Can you work these out from the drawing? Everything is in mm from the part's minimum corner. Give positions to 0.01 mm unless a question says otherwise; leave off trailing zeros. Order: outer loops, then holes, each group sorted by start corner. A loop starts at its lowest first (then second) coordinate and runs counter-clockwise, first axis right, second up. Notation, with made-up numbers: (8, 16.25) - (52, 16.25) arc R12 cw to (52, 36.25) - close; hole circle Ø4 at (13.5, 3.5). An arc over 180 degrees is marked (long way). Answer as a JSON object with one key per item and string values.
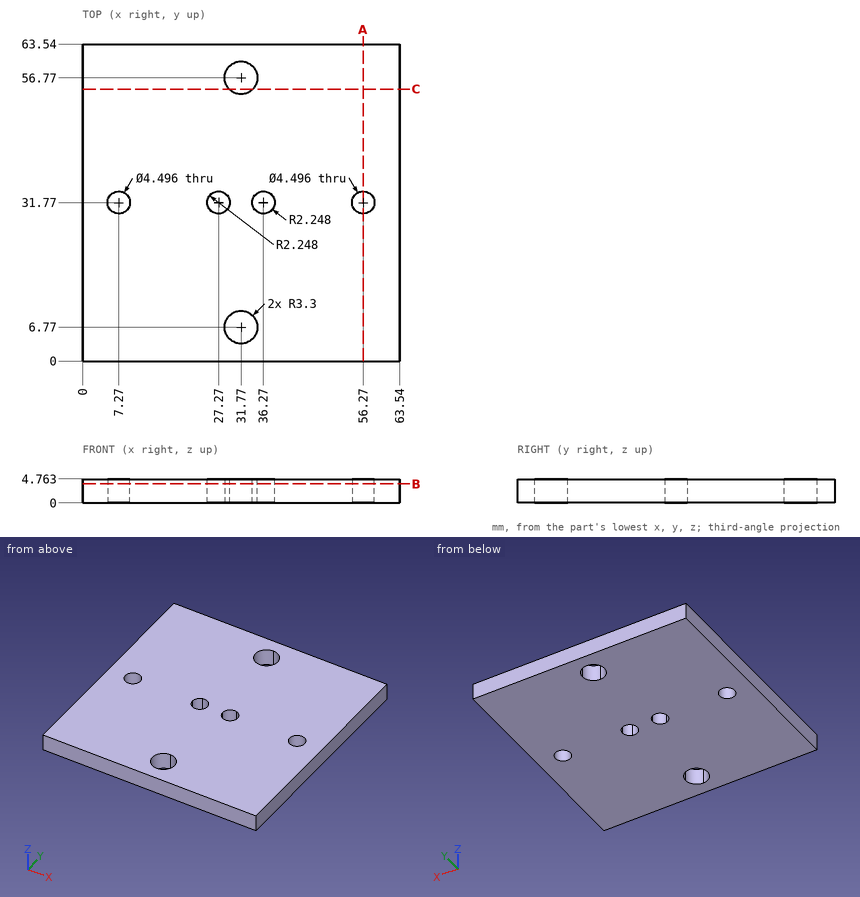
Q1. If we section it at C-C, the plane y = 54.5: Please give me the cut outline in (x, z) (1 decimal), then the cut area to 3 significant figures.
Recorded:
{"outline": "(0, 0) - (29.4, 0) - (29.4, 4.8) - (0, 4.8) - close; (34.2, 0) - (63.5, 0) - (63.5, 4.8) - (34.2, 4.8) - close", "area": "280 mm^2"}
Q2. I need wall thicknesses on L1, parallel to X at y = 31.77, z = 3.4; L2, parallel to Y at x = 7.27, z = 2.05; L3, parallel to X at y = 7, z = 2. Which ranges of each line are inside material? Lowest first, please.
Recorded:
{"L1": "x = 0 to 5.02, 9.52 to 25.02, 29.52 to 34.02, 38.52 to 54.02, 58.52 to 63.54", "L2": "y = 0 to 29.52, 34.02 to 63.54", "L3": "x = 0 to 28.48, 35.06 to 63.54"}
Q3. If we section it at A-A, the plane x = 56.27: Please give me the cut outline in (y, z).
Recorded:
{"outline": "(0, 0) - (29.52, 0) - (29.52, 4.76) - (0, 4.76) - close; (34.02, 0) - (63.54, 0) - (63.54, 4.76) - (34.02, 4.76) - close"}
Q4. I'm going to push flat-ended pins straight in: pin 1 Ø4 at (x, y) = (31, 23) entering from -Z; pin 2 Ø4 at (x, y) = (56.27, 31.77) entering from -Z. Where does each tip first touch, or does it pass through?
Recorded:
{"pin 1": "stops at z = 0", "pin 2": "passes through"}
Q5. If we section it at B-B, the plane z = 3.8: Count the separate pieces of the cut face and the enclosed holes in it, then the cut area to 3 significant figures.
Recorded:
{"separate pieces": "1", "enclosed holes": "6", "area": "3,910 mm^2"}
